```python
from build123d import *

# Parameters (mm, degrees)
F0_R      = 76.2
F1_DEPTH  = 69.596
F3_R      = 17.78
F4_DEPTH  = 159.004
F5_R      = 15.875
F6_DEPTH  = 258.064
F7_W      = 59.475604
F7_H      = 45.754954
F8_DEPTH  = 139.7
F9_W      = 33.02
F9_H      = 38.1
F10_DEPTH = 170.434
F11_W     = 20.298936
F11_H     = 62.223652
F12_DEPTH = 135.128
F13_R     = 16.35239
F14_DEPTH = 69.596
F16_DEPTH = 136.652


with BuildPart() as f1:
    # F0 (on Front) → F1 (new body, symmetric)
    with BuildSketch(Plane.XZ):
        Circle(F0_R)
    extrude(amount=F1_DEPTH, both=True)

    # F3 (on offset) → F4 (join)
    with BuildSketch(Plane.YZ.offset(79.756)):
        with Locations((-44.196, 0)):
            Circle(F3_R)
        Circle(F3_R)
        with Locations((44.196, 0)):
            Circle(F3_R)
    extrude(amount=-F4_DEPTH)

    # F5 (on offset) → F6 (cut)
    with BuildSketch(Plane.YZ.offset(79.756)):
        with Locations((-44.196, 0)):
            Circle(F5_R)
        Circle(F5_R)
        with Locations((44.196, 0)):
            Circle(F5_R)
    extrude(amount=-F6_DEPTH, mode=Mode.SUBTRACT)

    # F7 (on face) → F8 (join)
    with BuildSketch(Plane.XZ.offset(69.596)):
        Rectangle(F7_W, F7_H)
    extrude(amount=-F8_DEPTH)

    # F9 (on offset) → F10 (cut)
    with BuildSketch(Plane.YZ.offset(79.756)):
        with Locations((-36.83, 48.198743)):
            Rectangle(F9_W, F9_H)
        with Locations((36.83, 48.198743)):
            Rectangle(F9_W, F9_H)
    extrude(amount=-F10_DEPTH, mode=Mode.SUBTRACT)

    # F11 (on face) → F12 (join)
    with BuildSketch(Plane(origin=(0, 69.596, 0), x_dir=(-1, 0, 0), z_dir=(0, 1, 0))):
        with Locations((0, 44.409219)):
            Rectangle(F11_W, F11_H)
    extrude(amount=-F12_DEPTH)

    # F13 (on Front) → F14 (join, symmetric)
    with BuildSketch(Plane.XZ):
        with Locations((0, -67.743778)):
            Circle(F13_R)
    extrude(amount=F14_DEPTH, both=True)

    # F15 (on face) → F16 (cut, symmetric)
    with BuildSketch(Plane(origin=(0, -53.34, 0), x_dir=(-1, 0, 0), z_dir=(0, 1, 0))):
        Polygon((-32.835285, 45.658743), (-32.835285, 29.148743), (-22.216139, 29.148743), (-22.675285, 45.658743), align=None)
    extrude(amount=F16_DEPTH, both=True, mode=Mode.SUBTRACT)


solid = f1.part
```
The listing builds one solid part. Answer for the finished solid, in the listing's coordinates (mm). A direction names the side the tool comes from. Coordinates: 2 decimals unless noted, no trailing zeros. Write each loop counter-clockwise with the first axis right and the second up, starting at its lowest first coordinate (ties: lowest second). Pieces come first, ordered by that corner, then holes.
Q1. The mould has two halves that part along X. Classify faces 5 (the flat face through (-29.738, 44, 0)), 6 (the flat face through (28, -61, 45.659)), 7 (the flat face through (79.756, -7, 15)): released by +X, released by -X, zero draft, split by the parting line, or undercut.
Returned:
face 5: released by -X
face 6: undercut
face 7: released by +X
Q2. Section A-A, the plane y = 0 is taken. Write down the section's boundary in (x, z) (3 decimals), then the cut area to 3 significant figures.
Returned:
outline: (-79.248, -17.78) - (-74.097, -17.78) arc R76.2 ccw to (-14.773, -74.754) arc R16.352 ccw to (14.773, -74.754) arc R76.2 ccw to (74.097, -17.78) - (79.756, -17.78) - (79.756, -15.875) - (29.738, -15.875) - (29.738, 15.875) - (79.756, 15.875) - (79.756, 17.78) - (74.097, 17.78) arc R76.2 ccw to (-74.097, 17.78) - (-79.248, 17.78) - (-79.248, 15.875) - (-29.738, 15.875) - (-29.738, -15.875) - (-79.248, -15.875) - close; hole (22.216, 29.149) - (32.835, 29.149) - (32.835, 45.659) - (22.675, 45.659) - close
area: 15,400 mm2
Q3. Section B-B, the plane z = 32 is taken. Give the number of separate pieces and of enclosed holes in the cut face, then the cut area to 3 significant figures.
Returned:
separate pieces: 4
enclosed holes: 0
area: 10,700 mm2
Q4. Which of the six approach directions +Z, -Z, +X, -X, +Y, -Y give full straight-line access (tool end or side, diameter ignored) to faces 1 (the cylindrical face through (-0.258, -0.974, -84.094)), 2 (the flat face through (-33, 53.34, 44)), 3 (the flat face through (32.835, 0, 38)), 4 (the cylindrical face through (77.595, 26.433, 0.782))?
Returned:
face 1: -Z, +Y, -Y
face 2: -X
face 3: +Y, -Y
face 4: +X
Q5. Section D-D, the plane z = 62.5 is taken. Write down the section's boundary in (x, y), then the cut area to 3 significant figures.
Returned:
outline: (-43.59, -69.6) - (43.59, -69.6) - (43.59, -53.34) - (10.15, -53.34) - (10.15, -20.32) - (43.59, -20.32) - (43.59, 20.32) - (10.15, 20.32) - (10.15, 53.34) - (43.59, 53.34) - (43.59, 69.6) - (-43.59, 69.6) - (-43.59, 53.34) - (-10.15, 53.34) - (-10.15, 20.32) - (-43.59, 20.32) - (-43.59, -20.32) - (-10.15, -20.32) - (-10.15, -53.34) - (-43.59, -53.34) - close
area: 7,720 mm2
Q6. Section C-C, the plane x = -55 is taken. Write down the section's boundary in (y, z) (3 decimals).
Returned:
outline: (-69.596, -52.739) - (69.596, -52.739) - (69.596, 52.739) - (53.34, 52.739) - (53.34, 29.149) - (20.32, 29.149) - (20.32, 52.739) - (-20.32, 52.739) - (-20.32, 29.149) - (-53.34, 29.149) - (-53.34, 52.739) - (-69.596, 52.739) - close; hole circle Ø31.75 at (-44.196, 0); hole circle Ø31.75 at (0, 0); hole circle Ø31.75 at (44.196, 0)
Q7. Given P1, Ø19, axis at x = -46, z = 47.5, coming from the +Y side; P2, Ø10, axis at y = 7.5, z = -38.5, coming from the +X side; P3, Ø1, axis at y = 13, z = 38.5, coming from the +X side, each flat-ended and moving along its own axis, determine where each tip first touches the part or whether it passes through.
Returned:
P1: stops at y = 69.6
P2: stops at x = 68.44
P3: stops at x = 66.05
Q8. Find the intervals of material crossed by line 1 along X through (y, z) = (14, -6.5); line 2 along Y through (x, z) = (51, -32); line 3 along Z through (x, y) = (59.5, 0) (3 decimals), in increasing order.
Returned:
line 1: x = -29.74 to 29.74
line 2: y = -69.6 to 69.6
line 3: z = -47.605 to -15.875, 15.875 to 47.605
